Build history of the part. All positions in model axes, mm. Face numbers are marked on the shaded views. A direction names the side the tool comes from. Coordinates: 2 decimals unless noted, no trailing zeros. Order: outer loops, then holes, each group sorted by start corner. A loop starts at its lowest first (then second) coordinate and runs counter-clockwise, first axis right, second up. Notation, with made-up numbers: M 10,-10 L 29,-10 A25 ccw 29,23 Z; hole C 60,10 d1. An arc over 180 degrees is marked long. Write item = value, one per line. Start each with the question number.
Q1. Band-saw the part on A-A on x = 39.37. Write the cut outline in (y, z), plus the area to 3 significant figures.
Q2. 3-axis set-ups, long thin cutter, end or side, ignore diameter. For the marked faces 4 and 5: which of +Z, -Z, +X, -X, +Y, -Y reach the whole face in a straight line?
Q3. Band-saw the part on D-D on x = 26. Write the cut outline in (y, z), plus the area to 3 significant figures.
Q4. Pull direction X, two halves, no side cores. Call the marked faces 1, 2 and 3: released by +X, released by -X, zero draft, split by the parting line, or undercut.
Q5. Pin check, flat tips, straight feed: P1, Ø6, axis at x = 9.5, z = -16, coming from the -Y side; P2, Ø8, axis at x = 17, y = 16, coming from the -Z side; P3, Ø5.5, axis at x = 36.83, z = -15.54, coming from the +Y side. Stop position of each tip, or through.
Q6. Band-saw the part on C-C on z = -7. Write the cut outline in (x, y), plus the area to 3 significant figures.
Q7. Drill centre lines: probe 1 along Y at (x, z) = (3.81, -1.75); probe 2 along X at (y, z) = (19, -5); probe 3 along Y at (x, z) = (39, -2). Where is each one in solid material? Low to high.
Q8. Band-saw the part on B-B on y = 10.16. Write the cut outline in (x, z).
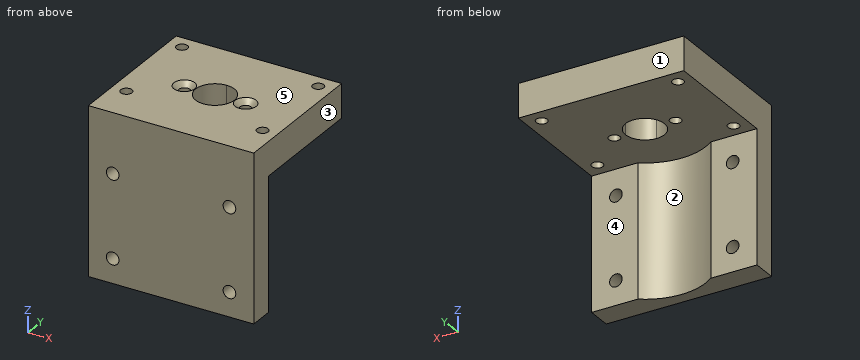
```python
from build123d import *

# Parameters (mm, degrees)
SKETCH1_W                                         = 43.18
SKETCH1_H                                         = 43.4848
SKETCH1_R                                         = 1.651
BASE_LEG_DEPTH                                    = 6.35
SKETCH3_R                                         = 2.286
PERPENDICULAR_LEG_DEPTH                           = 8.8138
CSK_FOR_M2_5_FLAT_HEAD_MACHINE_SCREW1_D           = 2.9
CSK_FOR_M2_5_FLAT_HEAD_MACHINE_SCREW1_CSINK_D     = 5.5
CSK_FOR_M2_5_FLAT_HEAD_MACHINE_SCREW1_CSINK_ANGLE = 90
SKETCH10_R                                        = 1.4605
HOLES_FOR_STABILIZING_THROUGH_SHAFT_DEPTH         = 68.217561998
SKETCH11_R                                        = 15.875
CUT_EXTRUDE1_DEPTH                                = 68.217561998


with BuildPart() as part:
    # Sketch1 → Base leg (new body)
    with BuildSketch(Plane(origin=(0, 0, 0), x_dir=(1, 0, 0), z_dir=(0, 1, 0))):
        with Locations((21.59, 21.7424)):
            Rectangle(SKETCH1_W, SKETCH1_H)
        with Locations(Location((6.35, 37.1348, 0), (0, 0, 270))):
            Circle(SKETCH1_R, mode=Mode.SUBTRACT)
        with Locations(Location((36.83, 37.1348, 0), (0, 0, 270))):
            Circle(SKETCH1_R, mode=Mode.SUBTRACT)
        with Locations(Location((36.83, 15.5448, 0), (0, 0, 270))):
            Circle(SKETCH1_R, mode=Mode.SUBTRACT)
        with Locations(Location((6.35, 15.5448, 0), (0, 0, 270))):
            Circle(SKETCH1_R, mode=Mode.SUBTRACT)
    extrude(amount=BASE_LEG_DEPTH)

    # Sketch3 → Perpendicular leg (add)
    # profile 1 of 3: a face of its own
    with BuildSketch(Plane.XY):
        with BuildLine():
            Line((0, 6.35), (21.59, 6.35))
            Line((21.59, 6.35), (21.59, 13.97))
            ThreePointArc((21.59, 13.97), (16.51, 19.05), (21.59, 24.13))
            Line((21.59, 24.13), (21.59, 38.1))
            Line((21.59, 38.1), (0, 38.1))
            Line((0, 38.1), (0, 6.35))
        make_face()
        with Locations((3.302, 19.05)):
            Circle(SKETCH3_R, mode=Mode.SUBTRACT)
    # profile 2 of 3: a face of its own
    with BuildSketch(Plane.XY):
        with Locations((3.302, 19.05)):
            Circle(SKETCH3_R)
    # profile 3 of 3: a face of its own
    with BuildSketch(Plane.XY):
        with BuildLine():
            Line((21.59, 13.97), (21.59, 6.35))
            Line((21.59, 6.35), (43.18, 6.35))
            Line((43.18, 6.35), (43.18, 38.1))
            Line((43.18, 38.1), (21.59, 38.1))
            Line((21.59, 38.1), (21.59, 24.13))
            ThreePointArc((21.59, 24.13), (25.182102448, 22.642102448), (26.67, 19.05))
            ThreePointArc((26.67, 19.05), (25.182102448, 15.457897552), (21.59, 13.97))
        make_face()
    extrude(amount=-PERPENDICULAR_LEG_DEPTH)

    # CSK for M2.5 Flat Head Machine Screw1 (through all)
    with Locations(Plane.XY):
        with Locations((13.5900033, 19.05), (29.5899967, 19.05)):
            CounterSinkHole(CSK_FOR_M2_5_FLAT_HEAD_MACHINE_SCREW1_D / 2, CSK_FOR_M2_5_FLAT_HEAD_MACHINE_SCREW1_CSINK_D / 2, counter_sink_angle=CSK_FOR_M2_5_FLAT_HEAD_MACHINE_SCREW1_CSINK_ANGLE)

    # Sketch10 → Holes for stabilizing through shaft (cut, through all)
    with BuildSketch(Plane(origin=(0, 0, -8.8138), x_dir=(-1, 0, 0), z_dir=(0, 0, -1))):
        with Locations((-39.37, 34.29)):
            Circle(SKETCH10_R)
        with Locations((-39.37, 10.16)):
            Circle(SKETCH10_R)
        with Locations((-3.81, 34.29)):
            Circle(SKETCH10_R)
        with Locations((-3.81, 10.16)):
            Circle(SKETCH10_R)
    extrude(amount=-HOLES_FOR_STABILIZING_THROUGH_SHAFT_DEPTH, mode=Mode.SUBTRACT)

    # Sketch11 → Cut-Extrude1 (cut, through all)
    with BuildSketch(Plane(origin=(0, 0, -8.8138), x_dir=(-1, 0, 0), z_dir=(0, 0, -1))):
        with Locations((-21.59, 19.05)):
            Circle(SKETCH11_R)
    extrude(amount=CUT_EXTRUDE1_DEPTH, mode=Mode.SUBTRACT)


solid = part.part
```
Recorded:
q1.outline = M 0,-43.48 L 6.35,-43.48 L 6.35,-8.81 L 8.7,-8.81 L 8.7,0 L 0,0 Z; M 11.62,-8.81 L 32.83,-8.81 L 32.83,0 L 11.62,0 Z; M 35.75,-8.81 L 38.1,-8.81 L 38.1,0 L 35.75,0 Z
q1.area = 504 mm2
q2.face_4 = -Z, +X, -X, +Y
q2.face_5 = +Z, +X, -X, +Y, -Y
q3.outline = M 0,-43.48 L 3.8,-43.48 L 3.8,-8.81 L 16.53,-8.81 L 16.53,0 L 0,0 Z; M 21.57,-8.81 L 38.1,-8.81 L 38.1,0 L 21.57,0 Z
q3.area = 423 mm2
q4.face_1 = zero draft
q4.face_2 = undercut
q4.face_3 = released by +X
q5.P1 = 0
q5.P2 = -8.81
q5.P3 = 6.35
q6.outline = M 0,0 L 43.18,0 L 43.18,38.1 L 0,38.1 Z; hole C 3.81,10.16 d2.92; hole C 3.81,34.29 d2.92; hole C 13.59,19.05 d2.9; hole C 21.59,19.05 d10.16; hole C 29.59,19.05 d2.9; hole C 39.37,10.16 d2.92; hole C 39.37,34.29 d2.92
q6.area = 1,520 mm2
q7.probe_1 = 0 to 8.7, 11.62 to 32.83, 35.75 to 38.1
q7.probe_2 = 0 to 12.14, 15.04 to 16.51, 26.67 to 28.14, 31.04 to 43.18
q7.probe_3 = 0 to 8.75, 11.57 to 32.88, 35.7 to 38.1
q8.outline = M 0,-8.81 L 2.35,-8.81 L 2.35,0 L 0,0 Z; M 5.27,-8.81 L 37.91,-8.81 L 37.91,0 L 5.27,0 Z; M 40.83,-8.81 L 43.18,-8.81 L 43.18,0 L 40.83,0 Z
